from build123d import *

# Parameters (mm, degrees)
SKETCH_1_R      = 51
EXTRUDE_1_DEPTH = 61
FILLET_1_R      = 5
SKETCH_6_W      = 41
SKETCH_6_H      = 41
SKETCH_7_W      = 0.25
SKETCH_7_H      = 45.977886119


with BuildPart() as part:
    # 草图1 → 凸台-拉伸1 (new body)
    with BuildSketch(Plane(origin=(0, 0, 0), x_dir=(1, 0, 0), z_dir=(0, 1, 0))):
        Circle(SKETCH_1_R)
    extrude(amount=EXTRUDE_1_DEPTH)

    # 圆角1
    fillet_1_edges = [part.edges().sort_by_distance(p)[0] for p in [
        (-51, 0, 0),
        (-51, 61, 0),
    ]]
    fillet(fillet_1_edges, radius=FILLET_1_R)

    # 草图6 → 切除-旋转4 (revolve, cut)
    with BuildSketch(Plane.XY):
        with Locations((20.5, 30.5)):
            Rectangle(SKETCH_6_W, SKETCH_6_H)
    revolve(axis=Axis((0, 0, 0), (0, 1, 0)), mode=Mode.SUBTRACT)

    # 草图7 → 切除-旋转5 (revolve, cut)
    with BuildSketch(Plane.XY):
        with Locations((-0.125, 38.011056941)):
            Rectangle(SKETCH_7_W, SKETCH_7_H)
    revolve(axis=Axis((0, 61, 0), (0, -1, 0)), mode=Mode.SUBTRACT)


solid = part.part
Could you check a few things on this model? Use its own coordinates, in mm. A direction names the side the tool comes from. Round coordinates to 2 decimals unless told otherwise and drop trailing zeros. Write each loop counter-clockwise with the first axis right and the second up, starting at its lowest first coordinate (ties: lowest second). Pieces come first, ordered by that corner, then holes. Notation, with made-up numbers: (40.5, 23) - (83.5, 23) arc R25 cw to (83.5, 36) - close; hole circle Ø3 at (-27.75, 23). An arc over 180 degrees is marked (long way). Put each result on its own line as item: value. Start each with the question number.
(1) Will these pins go through, and if not, where does the flat tip stop? pin 1 (10 mm diameter, centred on y = 15, z = -9, fed in from +X); pin 2 (5 mm diameter, centred on y = 7.5, z = 39, fed in from +X); pin 3 (4 mm diameter, centred on x = -6.5, y = 16, fed in from +Z); pin 4 (24.5 mm diameter, centred on x = -7.5, z = 14.5, fed in from -Y).
(2) I want a section at A-A, the plane y = 47. Please give me the cut outline in (x, z), plus the area to 3 significant figures.
(3) I need wall thicknesses on probe 1 along X at (y, z) = (22, 0); probe 2 along X at (y, z) = (55, 0). Which ranges of each line are inside material? Lowest first, please.
(4) For faces 1 (the flat face through (-1, 61, -1)), 2 (the flat face through (1, 51, -1)), which set-ups out of +Z, -Z, +X, -X, +Y, -Y let a thin tool reach every point of the face, with its end or its side?
(5) Thinking about a two-plate mould opening in Y: for faces 3 (the flat face through (-1, 0, -1)), 4 (the cylindrical face through (-11.056, 30.143, 49.787)), 5 (the cylindrical face through (-9, 31, 40)), 6 (the flat face through (1, 10, -1)), which applies, released by +Y, released by -Y, zero draft, split by the parting line, or undercut?
Here are the results:
1. pin 1: stops at x = 50.84
1. pin 2: stops at x = 35.62
1. pin 3: stops at z = 50.8
1. pin 4: stops at y = 0
2. outline: circle Ø102 at (0, 0); hole circle Ø82 at (0, 0)
2. area: 2,890 mm^2
3. probe 1: x = -51 to -41, 41 to 51
3. probe 2: x = -51 to -0.25, 0.25 to 51
4. face 1: +Z, -Z, +X, -X, +Y
4. face 2: none
5. face 3: released by -Y
5. face 4: zero draft
5. face 5: undercut
5. face 6: undercut
